Autodesk Inventor part; units mm, degrees
ref_plane "YZ Plane" through (0, 0, 0) normal (1, 0, 0) x (0, 1, 0)
ref_plane "XZ Plane" through (0, 0, 0) normal (0, 1, 0) x (-1, 0, 0)
ref_plane "XY Plane" through (0, 0, 0) normal (0, 0, 1) x (1, 0, 0)
sketch "Sketch1" plane through (0, 0, 0) normal (0, 1, 0) x (-1, 0, 0)
  line L0 (0, 0) -> (0, -6.3397)
  line L1 (0, -6.3397) -> (15, -15)
  line L2 (30, 0) -> (0, 0)
  line L3 (30, 0) -> (30, -15)
  line L4 (30, -15) -> (15, -15)
  dimension "d1" = 60
  dimension "d25" = 15
  dimension "d26" = 15
  dimension "d27" = 15
extrude "Extrusion1" add sketch "Sketch1" along normal blind 7
sketch "Sketch2" plane through (-15, 0, -15) normal (0.5, 0, -0.866) x (-0.866, 0, -0.5)
  line L0 (-17.3205, 0) -> (0, 0)
  line L1 (0, 0) -> (0, 7)
  line L2 (-17.3205, 7) -> (0, 7)
  line L3 (-17.3205, 0) -> (-17.3205, 7)
  circle A0 centre (-3.6603, 3.5) radius 1.45
  circle A1 centre (-13.6603, 3.5) radius 1.45
  point P0 (-20.4904, 0)
  dimension "d5" = 2.9
  dimension "d6" = 10
  dimension "d8" = 7
  dimension "d9" = 3.5
  dimension "d10" = 17.3205
  dimension "d11" = 3.6603
extrude "Extrusion2" cut sketch "Sketch2" against normal through all contours A0 | A1
sketch "Sketch6" plane through (0, 7, 0) normal (0, 1, 0) x (1, 0, 0)
  line L0 (0, 0) -> (0, 6.3397)
  line L1 (0, 6.3397) -> (-15, 15)
  line L2 (-15, 15) -> (-30, 15)
  line L3 (-30, 15) -> (-30, 0)
  line L4 (-30, 0) -> (0, 0)
  line L5 (0, 6.3397) -> (-15, 15)
  line L6 (-30, 0) -> (0, 0)
  line L7 (-25.5, 15) -> (-25.5, 0)
  dimension "d34" = 4.5
extrude "Extrusion5" add sketch "Sketch6" along normal blind 7 contours L4 L3 L2 L7
sketch "Sketch8" plane through (-25.5, 7, 0) normal (1, 0, 0) x (0, 0, -1)
  line L0 (15, 0) -> (0, 0)
  line L1 (15, 0) -> (15, 7)
  line L2 (0, 7) -> (15, 7)
  line L3 (0, 0) -> (0, 7)
  circle A0 centre (7.5, 3.5) radius 1.75
  point P0 (0, -7)
  point P1 (0, 3.5)
  point P2 (7.5, 0)
  dimension "d35" = 3.5
extrude "Extrusion7" cut sketch "Sketch8" against normal through all contours A0
equation "\"d9\" = 0.5 * d8"
equation "\"d11\" = -0.5 * d6 + 0.5 * d10"
properties part number "LEDBracket" material "ABS Plastic"
Model file for the job. Use its own axes, mm. A direction names the side the tool comes from. Coordinates: 2 decimals unless noted, no trailing zeros. Write each loop counter-clockwise with the first axis right and the second up, starting at its lowest first coordinate (ties: lowest second). Pieces come first, ordered by that corner, then holes. Notation, with made-up numbers: (2.25, 67) - (7.25, 67) arc R11 ccw to (7.25, 79) - close; hole circle Ø4 at (72, 32.5). An arc over 180 degrees is marked (long way). One line per item, written item: value. Start each with the question number.
1. Slice it at C-C (x = -25). Write the cut outline in (y, z).
2. Probe line 1 (Y direction, x = -27.6, z = -7.5); line 2 (X direction, y = 12.5, z = -10.5); line 3 (Y direction, x = -12, z = -9.25). List the from-to ranges inside material, lowest first. Write a range as from..to.
3. Slice it at D-D (z = -5). Count the separate pieces of the cut face and the enclosed holes in it, plus the area to 3 significant figures.
4. Flat gauge pins, fed straight in: pin 1 (4 mm diameter, centred on x = -21.5, y = 9.5, fed in from -Z); pin 2 (1 mm diameter, centred on y = 2.5, z = -7.5, fed in from +X); pin 3 (4.5 mm diameter, centred on x = -17.5, z = -5.5, fed in from +Y). Where does each tip first touch, or does it go through?
5. Slice it at A-A (y = 10.5). Write the cut outline in (x, z).
6. Mould opens along X. For faces 1 (the flat face through (-24, 5, -15)), 2 (the cylindrical face through (-6.9, 3.9, -4.5)), 3 (the flat face through (-7.4, 3.45, -10.61)) say: released by +X, released by -X, zero draft, split by the parting line, or undercut.
7. Slice it at B-B (y = 2.5). Write the cut outline in (x, z).
8. Tool access for faces 4 (the flat face through (-25.5, 9.7, -9.3)), 5 (the flat face through (-28, 14, -8)): list every direction of +Z, -Z, +X, -X, +Y, -Y with a clear straight run to the whole face (end or side of a thin tool).
Answers below:
1. outline: (0, -15) - (7, -15) - (7, 0) - (0, 0) - close
2. line 1: y = 0..8.75, 12.25..14
2. line 2: x = -30..-25.5
2. line 3: y = 0..7
3. separate pieces: 1
3. enclosed holes: 2
3. area: 226 mm^2
4. pin 1: passes through
4. pin 2: stops at x = -1.14
4. pin 3: stops at y = 7
5. outline: (-30, -15) - (-25.5, -15) - (-25.5, -9.25) - (-30, -9.25) - close; (-30, -5.75) - (-25.5, -5.75) - (-25.5, 0) - (-30, 0) - close
6. face 1: zero draft
6. face 2: undercut
6. face 3: released by +X
7. outline: (-30, -15) - (-15, -15) - (-12.74, -13.69) - (-20.65, 0) - (-30, 0) - close; (-18.22, 0) - (-10.92, -12.64) - (-4.08, -8.69) - (-9.1, 0) - close; (-6.67, 0) - (-2.26, -7.64) - (0, -6.34) - (0, 0) - close
8. face 4: +Z, -Z, +X, +Y
8. face 5: +Z, -Z, +X, -X, +Y
